Input: part model. Units: mm. Frame: model coordinates. Coordinates: 2 decimals unless noted, no trailing zeros. Write each question's results on one line, items separated by ' | '.
```python
from build123d import *

# Parameters (mm, degrees)
BOSS_EXTRU_1_DEPTH                                 = 960
ENL_V_MAT_EXTRU_1_DEPTH                            = 961.134334351
DIAM_TRE_DU_PER_AGE_0_4_0_4_1_D                    = 0.4
CHAMBRAGE_POUR_VIS_T_TE_HEXAGONALE_M41_D           = 4.5
CHAMBRAGE_POUR_VIS_T_TE_HEXAGONALE_M41_CBORE_D     = 8.5
CHAMBRAGE_POUR_VIS_T_TE_HEXAGONALE_M41_CBORE_DEPTH = 3.1
CONG_1_R                                           = 0.2
CONG_2_R                                           = 0.5
CONG_3_R                                           = 1
R_P_TITION_LIN_AIRE1_COUNT                         = 16
R_P_TITION_LIN_AIRE1_PITCH                         = 60


with BuildPart() as part:
    # Esquisse1 → Boss.-Extru.1 (new body)
    with BuildSketch(Plane.XZ):
        with BuildLine():
            Line((13.5, 3), (13.5, 8.7))
            Line((13.5, 8.7), (-13.5, 8.7))
            Line((-13.5, 8.7), (-13.5, 3))
            Line((-13.5, 3), (-7.8, 3))
            ThreePointArc((-7.8, 3), (-7.05, 2.25), (-7.8, 1.5))
            Line((-7.8, 1.5), (-11, 1.5))
            Line((-11, 1.5), (-11, 0))
            Line((-11, 0), (11, 0))
            Line((11, 0), (11, 1.5))
            Line((11, 1.5), (7.8, 1.5))
            ThreePointArc((7.8, 1.5), (7.05, 2.25), (7.8, 3))
            Line((7.8, 3), (13.5, 3))
        make_face()
    extrude(amount=-BOSS_EXTRU_1_DEPTH)

    # Esquisse2 → Enlèv. mat.-Extru.1 (cut, through all)
    with BuildSketch(Plane(origin=(0, 960, 0), x_dir=(-1, 0, 0), z_dir=(0, 1, 0))):
        Polygon((8.75, 8.7), (-8.75, 8.7), (-8.75, 7.6), (-12, 7.6), (-12, 4.1), (12, 4.1), (12, 7.6), (8.75, 7.6), align=None)
    extrude(amount=-ENL_V_MAT_EXTRU_1_DEPTH, mode=Mode.SUBTRACT)

    # Diamètre du perçage Ø0.4 (0.4)1 (through all)
    with Locations(Plane(origin=(0, 0, 0), x_dir=(-1, 0, 0), z_dir=(0, -1, 0))):
        with Locations((7.75, -4.1), (-7.75, -4.1)):
            Hole(DIAM_TRE_DU_PER_AGE_0_4_0_4_1_D / 2)

    # Chambrage pour vis à tête hexagonale M41 (through all)
    with Locations(Plane.XY.offset(4.1)):
        with Locations((0, 20), (0, 80)):
            chambrage_pour_vis_t_te_hexagonale_m41 = CounterBoreHole(CHAMBRAGE_POUR_VIS_T_TE_HEXAGONALE_M41_D / 2, CHAMBRAGE_POUR_VIS_T_TE_HEXAGONALE_M41_CBORE_D / 2, CHAMBRAGE_POUR_VIS_T_TE_HEXAGONALE_M41_CBORE_DEPTH)

    # Congé1
    cong_1_edges = [part.edges().sort_by_distance(p)[0] for p in [
        (11, 480, 1.5),
        (-11, 480, 1.5),
    ]]
    fillet(cong_1_edges, radius=CONG_1_R)

    # Congé2
    cong_2_edges = [part.edges().sort_by_distance(p)[0] for p in [
        (-12, 480, 7.6),
        (-12, 480, 4.1),
        (12, 480, 4.1),
        (12, 480, 7.6),
    ]]
    fillet(cong_2_edges, radius=CONG_2_R)

    # Congé3
    cong_3_edges = [part.edges().sort_by_distance(p)[0] for p in [
        (-13.5, 480, 3),
        (-13.5, 480, 8.7),
        (13.5, 480, 8.7),
        (13.5, 480, 3),
    ]]
    fillet(cong_3_edges, radius=CONG_3_R)

    # Répétition linéaire1: Chambrage pour vis à tête hexagonale M41 ×16
    with Locations(*[(0, i * R_P_TITION_LIN_AIRE1_PITCH, 0) for i in range(1, R_P_TITION_LIN_AIRE1_COUNT)]):
        add(chambrage_pour_vis_t_te_hexagonale_m41, mode=Mode.SUBTRACT)


solid = part.part
```
(1) Pin query (flat end, axial travel): P1, Ø0.5, axis at y = 584, z = 8, coming from the +X side; P2, Ø4, axis at x = -1, y = 380.5, coming from the +Z side; P3, Ø7.5, axis at x = -1, y = 272, coming from the +Z side; P4, Ø4, axis at x = -7, z = 6.5, coming from the +Y side. Return the tip coordinate at first contact, or that it passes through.
Return value:
P1: x = 13.5 | P2: z = 1 | P3: z = 4.1 | P4: through
(2) Line query: line 1 along Z through (x, y) = (-10.75, 838); line 2 along Z through (x, y) = (8.5, 98); line 3 along X through (y, z) = (320, 0.2). Output: solid intervals per line, ascending. Write a range as from..to.
Return value:
line 1: 0..1.5, 3..4.1, 7.6..8.7 | line 2: 0..1.5, 3..4.1 | line 3: -11..-2.25, 2.25..11
(3) Mould query, pull axis X, two halves, no side actions, for faces 1 (the face through (0, 487, 4.1)), 2 (the face through (0, 473, 0)). Classes: +X half, -X half, draft (parallel to the pull), parting line (faces both ways), or undercut.
Return value:
face 1: undercut | face 2: draft
